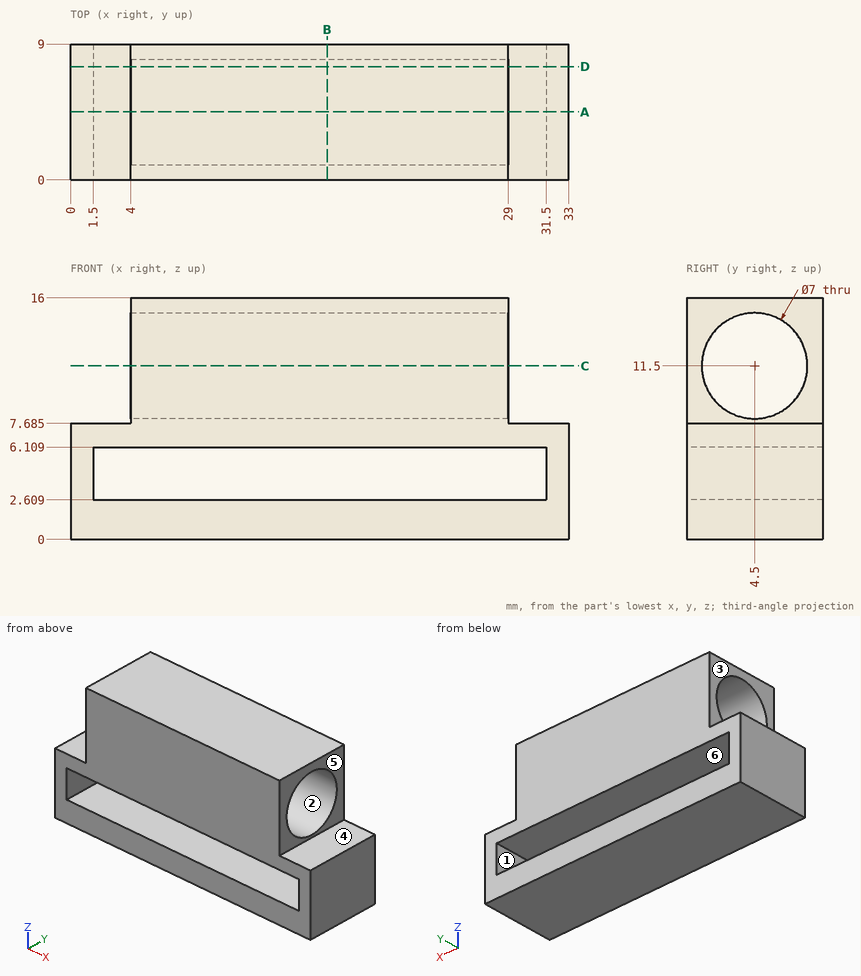
Could you check a few things on this drawing? It's one solid part, dimensions in mm from its lowest x, y, z. A direction names the side the tool comes from. Round coordinates to 2 decimals unless told otherwise and drop trailing zeros. Order: outer loops, then holes, each group sorted by start corner. A loop starts at its lowest first (then second) coordinate and runs counter-clockwise, first axis right, second up. Notation, with made-up numbers: M 38,-28 L 57,-28 A29 ccw 57,8 Z; hole C -37,63.25 d1. An arc over 180 degrees is marked long. One line per item, written item: value.
(1) Imagine slicing it at C-C (z = 11.5). Write out the boundary of the cut face in (x, y).
Ans:
outline: M 4,0 L 29,0 L 29,1 L 4,1 Z; M 4,8 L 29,8 L 29,9 L 4,9 Z
(2) I need wall thicknesses on line 1 along Y through (x, z) = (10.75, 11.5); line 2 along X through (y, z) = (4.5, 4.75); line 3 along Z through (x, y) = (8, 4.25). Which ranges of each line are inside material? Lowest first, please. Write a range as from..to.
Ans:
line 1: y = 0..1, 8..9
line 2: x = 0..1.5, 31.5..33
line 3: z = 0..2.61, 6.11..8.01, 14.99..16
(3) Which directions (+Z, -Z, +X, -X, +Y, -Y) give clear straight access to the entire face, cutting with the end or side of a thin tool? Please do the marked faces 1, 2 and 3.
Ans:
face 1: +Y, -Y
face 2: +X, -X
face 3: +Z, -X, +Y, -Y
(4) Imagine slicing it at D-D (y = 7.5). Write out the boundary of the cut face in (x, z) (1 decimal), and give its area (3 significant figures).
Ans:
outline: M 0,0 L 33,0 L 33,7.7 L 29,7.7 L 29,9.7 L 4,9.7 L 4,7.7 L 0,7.7 Z; M 4,13.3 L 29,13.3 L 29,16 L 4,16 Z; hole M 1.5,2.6 L 31.5,2.6 L 31.5,6.1 L 1.5,6.1 Z
area: 266 mm^2
(5) I'm going to push flat-ended pins straight in: P1, Ø2, axis at x = 1.5, y = 4, coming from the +Z side (3 decimals); P2, Ø4, axis at y = 3, z = 13.5, coming from the -X side. Where does each tip first touch, or does it pass through?
Ans:
P1: stops at z = 7.685
P2: stops at x = 4
(6) Imagine slicing it at A-A (y = 4.5). Write out the boundary of the cut face in (x, z) (3 decimals).
Ans:
outline: M 0,0 L 33,0 L 33,7.685 L 29,7.685 L 29,8 L 4,8 L 4,7.685 L 0,7.685 Z; M 4,15 L 29,15 L 29,16 L 4,16 Z; hole M 1.5,2.609 L 31.5,2.609 L 31.5,6.109 L 1.5,6.109 Z
(7) Imagine slicing it at B-B (x = 17). Write out the boundary of the cut face in (y, z).
Ans:
outline: M 0,0 L 9,0 L 9,2.61 L 0,2.61 Z; M 0,6.11 L 9,6.11 L 9,16 L 0,16 Z; hole C 4.5,11.5 d7
(8) If we mould it in two halves opening along X, with no side actions, what happens to the marked faces 4, 5 and 6? For each: released by +X, released by -X, zero draft, split by the parting line, or undercut.
Ans:
face 4: zero draft
face 5: released by +X
face 6: undercut
